from build123d import *


with BuildPart() as part:
    # Çizim1 → Döndür1 (revolve)
    with BuildSketch(Plane.XY, mode=Mode.PRIVATE) as d_nd_r1_sk:
        with BuildLine():
            Line((-25.497397444, 0), (-30.8, 0))
            ThreePointArc((-30.8, 0), (-30.941421356, 0.058578644), (-31, 0.2))
            Line((-31, 0.2), (-31, 13.8))
            Line((-31, 13.8), (-30.8, 14))
            Line((-30.8, 14), (-28.45, 14))
            Line((-28.45, 14), (-28.208094182, 13.804439517))
            Line((-28.208094182, 13.804439517), (-25.301836961, 0.241905818))
            ThreePointArc((-25.301836961, 0.241905818), (-25.341864226, 0.074264491), (-25.497397444, 0))
        make_face()
    revolve(d_nd_r1_sk.sketch.rotate(Axis((0, 0, 0), (0, 1, 0)), 270), axis=Axis((0, 0, 0), (0, 1, 0)))


solid = part.part
Work out the finished part from the listing and answer in its coordinate system (mm). Give positions to 0.01 mm unless a question says otherwise; leave off trailing zeros. Loops run counter-clockwise (first coordinate to the right, second up) from the corner with the lowest first, then second, coordinate; pieces in that order, holes last. Notation, with made-up numbers: (16, 63.25) -> (39, 63.25) arc R30 ccw to (39, 102.25) -> close; hole circle Ø1 at (-8.75, -9.75). An arc over 180 degrees is marked (long way). Use a Markdown table: item, result. Add a question column.
1. Section D-D on y = 11.25 is taken. Determine the outline of the cut face in (x, z).
2. Section A-A on z = 0 is taken. Determine the outline of the cut face in (x, y).
3. Find the intervals of material crossed by probe 1 along X at (y, z) = (7.75, -15); probe 2 along Z at (x, y) = (0.5, 8.75); probe 3 along Z at (x, y) = (-19, 11.75), in increasing order.
4. Flat-ended cylindrical pins translate along their axes: pin 1 Ø8 at (x, y) = (-15, 2.5) entering from -Z; pin 2 Ø4 at (y, z) = (1.5, 12) entering from +X; pin 3 Ø1 at (y, z) = (12.5, 14) entering from +X. Find the tip coordinate at first contact, or state that the pin passes through.
5. Section B-B on x = 0 is taken. Determine the outline of the cut face in (y, z).
6. Section C-C on y = 6.25 is taken. Determine the outline of the cut face in (x, z).
7. Determine the mould class of faces 1 (the conical face through (-25.226, 0.9, 3.312)), 2 (the flat face through (9, 14, -27.2)), 3 (the cylindrical face through (-30.736, 7.095, 4.036)) for opening direction Z: released by +Z, released by -Z, zero draft, split by the parting line, or undercut.
Results below:
| question | item | result |
|---|---|---|
| 1 | outline | circle Ø62 at (0, 0); hole circle Ø55.32 at (0, 0) |
| 2 | outline | (-31, 0.2) arc R0.2 ccw to (-30.8, 0) -> (-25.5, 0) arc R0.2 ccw to (-25.3, 0.24) -> (-28.21, 13.8) -> (-28.45, 14) -> (-30.8, 14) -> (-31, 13.8) -> close; (25.3, 0.24) arc R0.2 ccw to (25.5, 0) -> (30.8, 0) arc R0.2 ccw to (31, 0.2) -> (31, 13.8) -> (30.8, 14) -> (28.45, 14) -> (28.21, 13.8) -> close |
| 3 | probe 1 | x = -27.13 to -22.34, 22.34 to 27.13 |
| 3 | probe 2 | z = -31 to -27.12, 27.12 to 31 |
| 3 | probe 3 | z = -24.49 to -20.25, 20.25 to 24.49 |
| 4 | pin 1 | stops at z = -28.98 |
| 4 | pin 2 | stops at x = 29.34 |
| 4 | pin 3 | stops at x = 27.91 |
| 5 | outline | (0, -30.8) arc R0.2 ccw to (0.2, -31) -> (13.8, -31) -> (14, -30.8) -> (14, -28.45) -> (13.8, -28.21) -> (0.24, -25.3) arc R0.2 ccw to (0, -25.5) -> close; (0, 25.5) arc R0.2 ccw to (0.24, 25.3) -> (13.8, 28.21) -> (14, 28.45) -> (14, 30.8) -> (13.8, 31) -> (0.2, 31) arc R0.2 ccw to (0, 30.8) -> close |
| 6 | outline | circle Ø62 at (0, 0); hole circle Ø53.18 at (0, 0) |
| 7 | face 1 | undercut |
| 7 | face 2 | zero draft |
| 7 | face 3 | split by the parting line |
